Source: CAD feature listing. Evaluate the final solid. Frame: model axes, mm. Give positions to 0.01 mm unless a question says otherwise; leave off trailing zeros. Order: outer loops, then holes, each group sorted by start corner. A loop starts at its lowest first (then second) coordinate and runs counter-clockwise, first axis right, second up. Notation, with made-up numbers: (-21.75, 84.25) - (-10.75, 84.25) arc R23 cw to (-10.75, 113.25) - close; hole circle Ø1 at (82.5, -8.5). An arc over 180 degrees is marked (long way). Write each question's results on one line, items separated by ' | '. Start each with the question number.
Item 1: Mould query, pull axis Y, two halves, no side actions, for faces 1 (the cylindrical face through (-3.047, -0.134, -0.032)), 2 (the cylindrical face through (-1.08, 4.88, -0.03)). Classes: released by +Y, released by -Y, zero draft, split by the parting line, or undercut.
Item 2: Contact query for flat-ended pins moving along their axis: pin 1 Ø3 at (y, z) = (2.5, -1) entering from +X; pin 2 Ø3.5 at (x, y) = (0, 0) entering from -Z; pin 3 Ø1.5 at (x, z) = (4, -1) entering from +Y; pin 4 Ø3 at (y, z) = (3, 1.5) entering from -X. Output: stop coordinate, or through.
Item 3: Line query: line 1 along X through (y, z) = (0, -0.35); line 2 along Y through (x, z) = (-1, -1.1). Output: solid intervals per line, ascending.
Item 4: Section C-C on z = -0.7. Output: boundary loops of the cut face in (x, y).
Item 5: Section A-A on x = 0. Output: boundary loops of the cut face in (y, z), and give its area (3 significant figures).
Autodesk Inventor part; units mm, degrees
ref_plane "YZ Plane" through (0, 0, 0) normal (1, 0, 0) x (0, 1, 0)
ref_plane "XZ Plane" through (0, 0, 0) normal (0, 1, 0) x (-1, 0, 0)
ref_plane "XY Plane" through (0, 0, 0) normal (0, 0, 1) x (1, 0, 0)
sketch "Skizze2" plane through (0, 0, 0) normal (0, 0, 1) x (1, 0, 0)
  line L0 (-7, 0) -> (7, 0)
  line L1 (0, 7) -> (0, -7)
  circle A0 centre (0, 0) radius 5
  circle A1 centre (0, 0) radius 3.05
  dimension "d13" = 10
  dimension "d14" = 6.1
extrude "Grundkörper" add sketch "Skizze2" along normal mid plane 5 contours A1 L1 A0 L0 | L0 A0 L1 A1 | A1 L0 A0 L1 | L1 A0 L0 A1
chamfer "Fase_Allgemein" distance 0.2 angle 45 4 edges at (-3.05, 0, 2.5) (-5, 0, 2.5) (-3.05, 0, -2.5) (-5, 0, -2.5)
properties part number "200-60-DIFFERENTIAL-BAR-04" material "Edelstahl"
Evaluation:
1) face 1: undercut | face 2: split by the parting line
2) pin 1: stops at x = 4.9 | pin 2: passes through | pin 3: stops at y = 3.8 | pin 4: stops at x = -4.77
3) line 1: x = -5 to -3.05, 3.05 to 5 | line 2: y = -4.9 to -2.88, 2.88 to 4.9
4) outline: circle Ø10 at (0, 0); hole circle Ø6.1 at (0, 0)
5) outline: (-5, -2.3) - (-4.8, -2.5) - (-3.25, -2.5) - (-3.05, -2.3) - (-3.05, 2.3) - (-3.25, 2.5) - (-4.8, 2.5) - (-5, 2.3) - close; (3.05, -2.3) - (3.25, -2.5) - (4.8, -2.5) - (5, -2.3) - (5, 2.3) - (4.8, 2.5) - (3.25, 2.5) - (3.05, 2.3) - close | area: 19.3 mm^2
